```python
from build123d import *

# Parameters (mm, degrees)
BOSS_EXTRUDE1_DEPTH = 17.1
FILLET1_R           = 10
SKETCH5_R           = 1.625
CUT_EXTRUDE1_DEPTH  = 21.5
BOSS_EXTRUDE2_DEPTH = 3


with BuildPart() as part:
    # Sketch1 → Boss-Extrude1 (new body, symmetric)
    with BuildSketch(Plane.XY):
        Polygon((-5.5, 17), (-3.5, 17), (-3.5, 1), (3.5, 1), (3.5, 17), (5.5, 17), (5.5, 1), (15, 1), (15, -1), (-15, -1), (-15, 1), (-5.5, 1), align=None)
    extrude(amount=BOSS_EXTRUDE1_DEPTH, both=True)

    # Fillet1
    fillet1_edges = [part.edges().sort_by_distance(p)[0] for p in [
        (-4.5, 17, -17.1),
        (4.5, 17, -17.1),
        (4.5, 17, 17.1),
        (-4.5, 17, 17.1),
    ]]
    fillet(fillet1_edges, radius=FILLET1_R)

    # Sketch5 → Cut-Extrude1 (cut, through all)
    with BuildSketch(Plane.ZY.offset(5.5)):
        with Locations((-9.1, 9)):
            Circle(SKETCH5_R)
        with Locations((9.1, 9)):
            Circle(SKETCH5_R)
    extrude(amount=-CUT_EXTRUDE1_DEPTH, mode=Mode.SUBTRACT)

    # Sketch7 → Boss-Extrude2 (add)
    with BuildSketch(Plane.XZ.offset(1)):
        Polygon((-15, 8), (-7.5, 16.6), (0, 8), (7.5, 16.6), (15, 8), (15, 2), (7.5, 10.6), (0, 2), (-7.5, 10.6), (-15, 2), align=None)
        Polygon((-15, -2), (-7.5, -10.6), (0, -2), (7.5, -10.6), (15, -2), (15, -8), (7.5, -16.6), (0, -8), (-7.5, -16.6), (-15, -8), align=None)
    extrude(amount=BOSS_EXTRUDE2_DEPTH)


solid = part.part
```
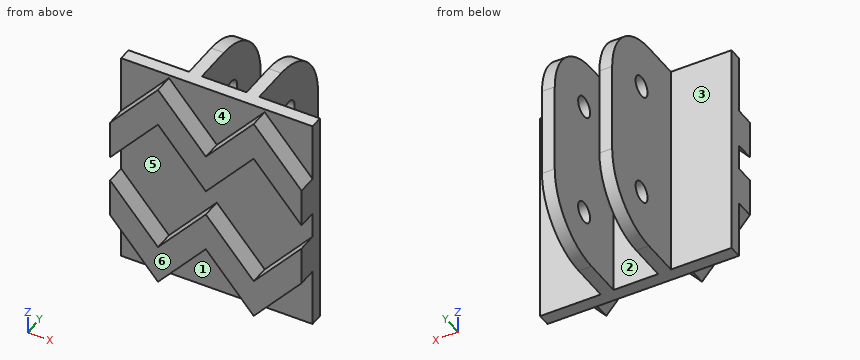
The model under review builds one solid part; all positions refer to its coordinate system, in mm. Face numbers are marked on the shaded views. A direction names the side the tool comes from. Round coordinates to 2 decimals unless told otherwise and drop trailing zeros. Loops run counter-clockwise (first coordinate to the right, second up) from the corner with the lowest first, then second, coordinate; pieces in that order, holes last.
1) Clearance check with flat-ended pins moving along their axes: P1, Ø8, axis at y = 6, z = -3.5, coming from the +X side; P2, Ø5, axis at x = 9.5, z = 1, coming from the +Y side; P3, Ø8, axis at y = 12.5, z = 3.5, coming from the -X side; P4, Ø3, axis at y = 9, z = -9.1, coming from the +X side. State where each tip first meets the part, or that it passes through.
Values follow:
P1: stops at x = 5.5
P2: stops at y = 1
P3: stops at x = -5.5
P4: passes through
2) The part is to be moulded in two halves that separate along Z. For the marked faces 5 and 6, say which applies: pulls with the +Z half, pulls with the -Z half, needs draft (parallel to the pull), parting line crosses it, or undercut.
Values follow:
face 5: undercut
face 6: needs draft
3) Consider section D-D on x = -2.5. State the section outline as (y, z) points, then the cut area to 3 significant figures.
Values follow:
outline: (-4, -10.87) - (-1, -10.87) - (-1, -17.1) - (1, -17.1) - (1, 17.1) - (-1, 17.1) - (-1, 10.87) - (-4, 10.87) - (-4, 4.87) - (-1, 4.87) - (-1, -4.87) - (-4, -4.87) - close
area: 104 mm2
4) Consider section C-C on y = 13.75. State the section outline as (x, z) points.
Values follow:
outline: (-5.5, -14.48) - (-3.5, -14.48) - (-3.5, 14.48) - (-5.5, 14.48) - close; (3.5, -14.48) - (5.5, -14.48) - (5.5, 14.48) - (3.5, 14.48) - close
5) Tool access review of the marked faces 1, 2, 3 and 4: name each direction out of +Z, -Z, +X, -X, +Y, -Y from which nothing blocks a thin tool from reaching the whole face with its end or side.
Values follow:
face 1: -Z, -Y
face 2: +Z, -Z, +Y
face 3: +Z, -Z, -X, +Y
face 4: +Z, -Y
6) Consider section B-B on z = -5. State the section outline as (x, y) points.
Values follow:
outline: (-15, -4) - (-12.38, -4) - (-12.38, -1) - (-2.62, -1) - (-2.62, -4) - (2.62, -4) - (2.62, -1) - (12.38, -1) - (12.38, -4) - (15, -4) - (15, 1) - (5.5, 1) - (5.5, 17) - (3.5, 17) - (3.5, 1) - (-3.5, 1) - (-3.5, 17) - (-5.5, 17) - (-5.5, 1) - (-15, 1) - close
7) Wall thickness on line 1 along X through (y, z) = (-1.25, 10.5); line 2 along X through (y, z) = (6.5, -16); line 3 along X through (y, z) = (-2, -16): over which ranges is each line inside the solid? List them lowest first.
Values follow:
line 1: x = -12.82 to -7.59, -7.41 to -2.18, 2.18 to 7.41, 7.59 to 12.82
line 2: x = -5.5 to -3.5, 3.5 to 5.5
line 3: x = -8.02 to -6.98, 6.98 to 8.02
8) Consider section A-A on y = 9. State the section outline as (x, z) points (3 decimals).
Values follow:
outline: (-5.5, -16.898) - (-3.5, -16.898) - (-3.5, -10.725) - (-5.5, -10.725) - close; (-5.5, -7.475) - (-3.5, -7.475) - (-3.5, 7.475) - (-5.5, 7.475) - close; (-5.5, 10.725) - (-3.5, 10.725) - (-3.5, 16.898) - (-5.5, 16.898) - close; (3.5, -16.898) - (5.5, -16.898) - (5.5, -10.725) - (3.5, -10.725) - close; (3.5, -7.475) - (5.5, -7.475) - (5.5, 7.475) - (3.5, 7.475) - close; (3.5, 10.725) - (5.5, 10.725) - (5.5, 16.898) - (3.5, 16.898) - close
